```python
from build123d import *

# Parameters (mm, degrees)
F0_W     = 38.1
F0_H     = 25.4
F1_DEPTH = 12.7
F3_DEPTH = 25.401
F4_W     = 12.529509142
F4_H     = 12.7
F4_W_2   = 13.1820067763
F5_DEPTH = 25.401
F6_W     = 12.4995596707
F6_H     = 13.7623953633
F7_DEPTH = 12.7
F8_R     = 6.780247306
F9_DEPTH = 12.701


with BuildPart() as f1:
    # F0 (on Front) → F1 (new body, symmetric)
    with BuildSketch(Plane.XZ):
        with Locations((19.05, 12.7)):
            Rectangle(F0_W, F0_H)
    extrude(amount=F1_DEPTH, both=True)

    # F2 (on face) → F3 (cut, through all)
    with BuildSketch(Plane.XZ.offset(12.7)):
        with BuildLine():
            Line((38.1, 25.4), (25.0590182841, 25.4))
            ThreePointArc((25.0590182841, 25.4), (37.7590182841, 12.7), (25.0590182841, 0))
            Line((25.0590182841, 0), (38.1, 0))
            Line((38.1, 0), (38.1, 25.4))
        make_face()
    extrude(amount=-F3_DEPTH, mode=Mode.SUBTRACT)

    # F4 (on face) → F5 (cut, through all)
    with BuildSketch(Plane.XY.offset(25.4)):
        with Locations((18.7942637131, -6.35)):
            Rectangle(F4_W, F4_H)
        with Locations((31.6500216722, -6.35)):
            Rectangle(F4_W_2, F4_H)
    extrude(amount=-F5_DEPTH, mode=Mode.SUBTRACT)

    # F6 (on face) → F7 (cut)
    with BuildSketch(Plane.XZ.offset(12.7)):
        with Locations((6.2497798353, 12.8240382764)):
            Rectangle(F6_W, F6_H)
    extrude(amount=-F7_DEPTH, mode=Mode.SUBTRACT)

    # F8 (on face) → F9 (cut, through all)
    with BuildSketch(Plane.XZ):
        with Locations((26.0712560266, 12.6046799123)):
            Circle(F8_R)
    extrude(amount=-F9_DEPTH, mode=Mode.SUBTRACT)


solid = f1.part
```
Check sheet for the modelled part. Datum: model origin and axes. Units: mm. A direction names the side the tool comes from. Round coordinates to 2 decimals unless told otherwise and drop trailing zeros. Loops run counter-clockwise (first coordinate to the right, second up) from the corner with the lowest first, then second, coordinate; pieces in that order, holes last. Notation, with made-up numbers: (83.5, 82) -> (125.5, 82) arc R20 cw to (125.5, 96) -> close; hole circle Ø3 at (38, 26). An arc over 180 degrees is marked (long way). Write item = value, one per line. Start each with the question number.
1) Gauge pin test, flat ends, axial feed: pin 1 Ø10 at (y, z) = (-6.5, 18) entering from +X; pin 2 Ø1.5 at (y, z) = (-2.5, 14.5) entering from -X; pin 3 Ø6 at (x, z) = (8.5, 9.5) entering from -Y; pin 4 Ø1.5 at (x, y) = (26.5, -2.5) entering from +Z. Record the tip position at first contact, or that the pin passes through.
2) Sectioned sample at B-B, the plane y = -4.75. Record the cut outline in (x, z).
3) Release check for a two-part mould opening along Z. For faces 4 (the flat face through (10, 3, 25.4)), 5 (the flat face through (6, -6, 5.943)), 6 (the flat face through (14, 12.7, 13)) record: released by +Z, released by -Z, zero draft, split by the parting line, or undercut.
4) Thickness scan on probe 1 along X at (y, z) = (4.5, 12.75); probe 2 along Y at (x, z) = (5.5, 18.25); probe 3 along Z at (x, y) = (21, 10.75). Record the ranges inside material, lowest first.
5) Set-up check for faces 1 (the flat face through (6, -12.7, 21)), 2 (the flat face through (6, -6, 19.705)), 3 (the flat face through (20, 0, 16)): record each of +Z, -Z, +X, -X, +Y, -Y from which the full face is reachable in a straight line by a thin tool's end or side.
6) Sectioned sample at C-C, the plane x = 21.5. Record the cut outline in (y, z).
Results are:
q1.pin_1 = 12.53
q1.pin_2 = 12.5
q1.pin_3 = 0
q1.pin_4 = through
q2.outline = (0, 0) -> (12.53, 0) -> (12.53, 25.4) -> (0, 25.4) -> (0, 19.71) -> (12.5, 19.71) -> (12.5, 5.94) -> (0, 5.94) -> close
q3.face_4 = released by +Z
q3.face_5 = undercut
q3.face_6 = zero draft
q4.probe_1 = 0 to 19.29, 32.85 to 37.76
q4.probe_2 = 0 to 12.7
q4.probe_3 = 0 to 8.1, 17.11 to 25.4
q5.face_1 = +Z, -Z, +X, -X, -Y
q5.face_2 = -X, -Y
q5.face_3 = +Z, -Z, +X, -Y
q6.outline = (0, 0) -> (12.7, 0) -> (12.7, 7.6) -> (0, 7.6) -> close; (0, 17.61) -> (12.7, 17.61) -> (12.7, 25.4) -> (0, 25.4) -> close
